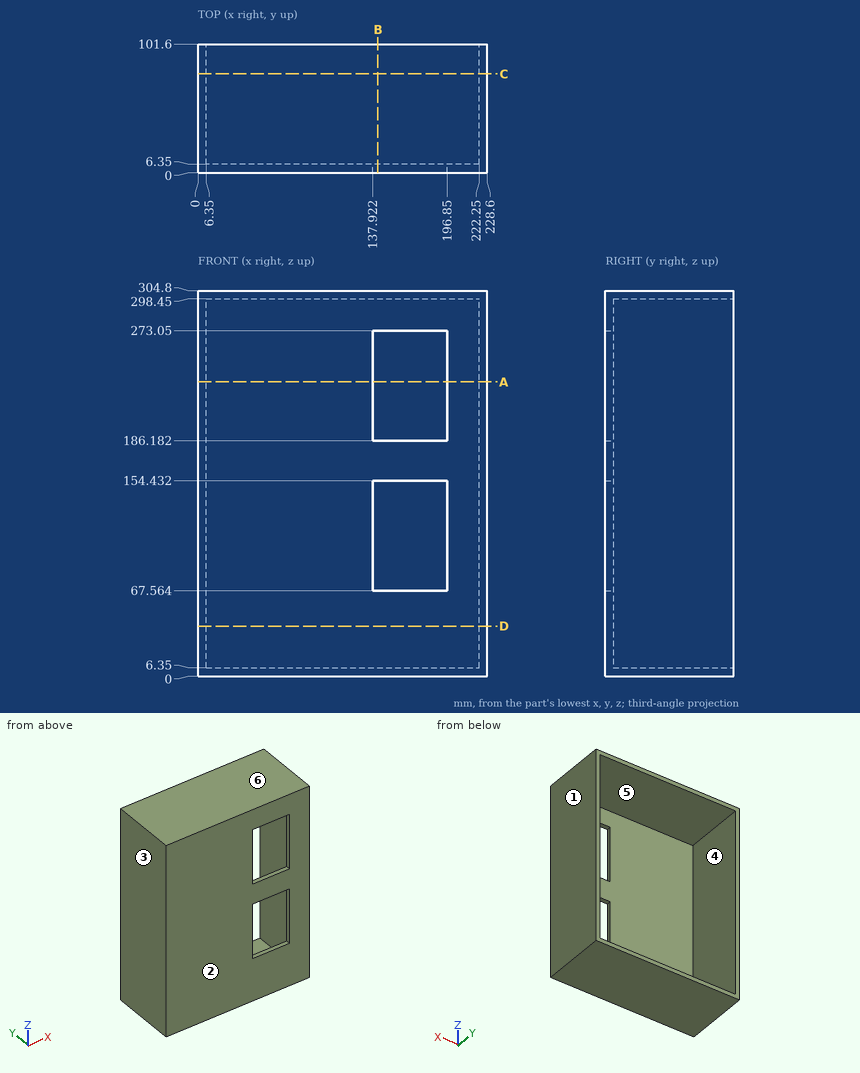
Check sheet for the drawn part. Datum: minimum x, y, z corner. Units: mm. A direction names the side the tool comes from. Coordinates: 2 decimals unless noted, no trailing zeros. Order: outer loops, then holes, each group sorted by start corner. A loop starts at its lowest first (then second) coordinate and runs counter-clockwise, first axis right, second up. Notation, with made-up numbers: (-11, 42.25) - (15, 42.25) arc R21 ccw to (15, 58.25) - close; hole circle Ø7 at (-36.75, 6.5). An arc over 180 degrees is marked (long way). Return JSON: item names as keys, results as strings.
(1) Go/stop test with a flat-tipped pin: pin 1 (6 mm diameter, centred on x = 36.5, z = 199, fed in from +Y). Record where the tip stops, or that it passes through.
Filled sheet:
{"pin 1": "stops at y = 6.35"}
(2) Mould release check, pull along X, two halves, no side actions. Record for the marked faces 1, 2, 3 and 4: pulls with the +X half, pulls with the -X half, needs draft (parallel to the pull), parting line crosses it, or undercut.
Filled sheet:
{"face 1": "pulls with the +X half", "face 2": "needs draft", "face 3": "pulls with the -X half", "face 4": "undercut"}
(3) Section check D-D, the plane z = 39.5. Record the cut outline in (x, y).
Filled sheet:
{"outline": "(0, 0) - (228.6, 0) - (228.6, 101.6) - (222.25, 101.6) - (222.25, 6.35) - (6.35, 6.35) - (6.35, 101.6) - (0, 101.6) - close"}
(4) Section check C-C, the plane y = 78. Record the cut outline in (x, z), and give its area (3 significant figures).
Filled sheet:
{"outline": "(0, 0) - (228.6, 0) - (228.6, 304.8) - (0, 304.8) - close; hole (6.35, 6.35) - (222.25, 6.35) - (222.25, 298.45) - (6.35, 298.45) - close", "area": "6,610 mm^2"}
(5) Thickness scan on line 1 along X through (y, z) = (55.5, 59); line 2 along Z through (x, y) = (182, 33); line 3 along Y through (x, z) = (135.5, 227.5). Record the ranges inside material, lowest first.
Filled sheet:
{"line 1": "x = 0 to 6.35, 222.25 to 228.6", "line 2": "z = 0 to 6.35, 298.45 to 304.8", "line 3": "y = 0 to 6.35"}
(6) Section check A-A, the plane z = 232.5. Record the cut outline in (x, y).
Filled sheet:
{"outline": "(0, 0) - (137.92, 0) - (137.92, 6.35) - (6.35, 6.35) - (6.35, 101.6) - (0, 101.6) - close; (196.85, 0) - (228.6, 0) - (228.6, 101.6) - (222.25, 101.6) - (222.25, 6.35) - (196.85, 6.35) - close"}
(7) Section check B-B, the plane x = 142. Record the cut outline in (y, z), and give its area (3 significant figures).
Filled sheet:
{"outline": "(0, 0) - (101.6, 0) - (101.6, 6.35) - (6.35, 6.35) - (6.35, 67.56) - (0, 67.56) - close; (0, 154.43) - (6.35, 154.43) - (6.35, 186.18) - (0, 186.18) - close; (0, 273.05) - (6.35, 273.05) - (6.35, 298.45) - (101.6, 298.45) - (101.6, 304.8) - (0, 304.8) - close", "area": "2,040 mm^2"}
(8) Access from +Z, -Z, +X, -X, +Y, -Y to the whole of each face (thin tool, end or side, straight path). Record for the marked faces 5 and 6.
Filled sheet:
{"face 5": "+Y", "face 6": "+Z, +X, -X, +Y, -Y"}
